Geometry check sheet. Reference: the model listing, model coordinates, mm. A direction names the side the tool comes from. Give positions to 0.01 mm unless a question says otherwise; leave off trailing zeros. Loops run counter-clockwise (first coordinate to the right, second up) from the corner with the lowest first, then second, coordinate; pieces in that order, holes last. Notation, with made-up numbers: (-30.75, -12) - (-15.75, -12) arc R22 ccw to (-15.75, 9) - close; hole circle Ø4 at (24, 54.25). An arc over 180 degrees is marked (long way). One line per question, with ' | ' between items. Start each with the question number.
from build123d import *

# Parameters (mm, degrees)
BOSS_EXTRUDE1_DEPTH = 13.125
SKETCH2_R           = 7
CUT_EXTRUDE1_DEPTH  = 106.5
SKETCH2_4_R         = 11.125
SKETCH2_4_R_2       = 7
CUT_EXTRUDE2_DEPTH  = 7
SKETCH4_R           = 4
BOSS_EXTRUDE3_DEPTH = 10
SKETCH5_R           = 6.5
BOSS_EXTRUDE4_DEPTH = 1
CIRPATTERN1_COUNT   = 2
CIRPATTERN1_ANGLE   = 45
SKETCH9_R           = 4
BOSS_EXTRUDE6_DEPTH = 20
CUT_EXTRUDE6_REACH  = 96.758
SKETCH10_R          = 1.5
SKETCH11_R          = 6.5
BOSS_EXTRUDE7_DEPTH = 13.5
SKETCH12_R          = 4
BOSS_EXTRUDE8_DEPTH = 13.75
SKETCH13_R          = 1.5
CUT_EXTRUDE7_DEPTH  = 13.75
SKETCH14_R          = 11.125
CUT_EXTRUDE8_DEPTH  = 17
SKETCH15_R          = 7
CUT_EXTRUDE9_DEPTH  = 1
SKETCH16_R          = 1.55
CUT_EXTRUDE10_DEPTH = 93.310955607


with BuildPart() as part:
    # Sketch1 → Boss-Extrude1 (new, symmetric)
    with BuildSketch(Plane(origin=(0, 0, 0), x_dir=(1, 0, 0), z_dir=(0, 1, 0))):
        Polygon((-49.25, 13.125), (-49.25, -13.125), (-49.25, -20.400017947), (-20.400017947, -49.25), (20.400017947, -49.25), (49.25, -20.400017947), (49.25, -13.125), (49.25, 13.125), (57.25, 13.125), (57.25, -23.713726446), (23.713726446, -57.25), (-23.713726446, -57.25), (-57.25, -23.713726446), (-57.25, 13.125), align=None)
    extrude(amount=BOSS_EXTRUDE1_DEPTH, both=True)

    # Sketch2 → Cut-Extrude1 (cut)
    with BuildSketch(Plane.ZY.offset(57.25)):
        with BuildLine():
            Line((-13.125, 13.125), (-13.125, 0))
            ThreePointArc((-13.125, 0), (-12.924585281, 2.284889562), (-12.329461667, 4.5))
            ThreePointArc((-12.329461667, 4.5), (-7.523400993, 10.7547228), (0, 13.125))
            Line((0, 13.125), (-13.125, 13.125))
        make_face()
        with BuildLine():
            ThreePointArc((-12.329461667, -4.5), (-12.924585281, -2.284889562), (-13.125, 0))
            Line((-13.125, 0), (-13.125, -13.125))
            Line((-13.125, -13.125), (0, -13.125))
            ThreePointArc((0, -13.125), (-7.523400993, -10.7547228), (-12.329461667, -4.5))
        make_face()
        Circle(SKETCH2_R)
        with BuildLine():
            ThreePointArc((-5.361902647, -4.5), (-6.577739678, -2.394439545), (-7, 0))
            Line((-7, 0), (-11.125, 0))
            ThreePointArc((-11.125, 0), (-10.88472093, -2.299668513), (-10.174262873, -4.5))
            Line((-10.174262873, -4.5), (-5.361902647, -4.5))
        make_face()
        with BuildLine():
            Line((-11.125, 0), (-7, 0))
            ThreePointArc((-7, 0), (-6.577739678, 2.394439545), (-5.361902647, 4.5))
            Line((-5.361902647, 4.5), (-10.174262873, 4.5))
            ThreePointArc((-10.174262873, 4.5), (-10.88472093, 2.299668513), (-11.125, 0))
        make_face()
        with BuildLine():
            ThreePointArc((-10.174262873, -4.5), (-10.88472093, -2.299668513), (-11.125, 0))
            Line((-11.125, 0), (-13.125, 0))
            ThreePointArc((-13.125, 0), (-12.924585281, -2.284889562), (-12.329461667, -4.5))
            Line((-12.329461667, -4.5), (-10.174262873, -4.5))
        make_face()
        with BuildLine():
            Line((-13.125, 0), (-11.125, 0))
            ThreePointArc((-11.125, 0), (-10.88472093, 2.299668513), (-10.174262873, 4.5))
            Line((-10.174262873, 4.5), (-12.329461667, 4.5))
            ThreePointArc((-12.329461667, 4.5), (-12.924585281, 2.284889562), (-13.125, 0))
        make_face()
    cut_extrude1 = extrude(amount=-CUT_EXTRUDE1_DEPTH, mode=Mode.SUBTRACT)

    # Sketch2_4 → Cut-Extrude2 (cut)
    with BuildSketch(Plane.ZY.offset(57.25)):
        Circle(SKETCH2_4_R)
        Circle(SKETCH2_4_R_2, mode=Mode.SUBTRACT)
    cut_extrude2 = extrude(amount=-CUT_EXTRUDE2_DEPTH, mode=Mode.SUBTRACT)

    # Mirror1: Cut-Extrude1, Cut-Extrude2 across plane
    add(cut_extrude1.mirror(Plane(origin=(0, 0, 0), x_dir=(0, 0, 1), z_dir=(1, 0, 0))), mode=Mode.SUBTRACT)
    add(cut_extrude2.mirror(Plane(origin=(0, 0, 0), x_dir=(0, 0, 1), z_dir=(1, 0, 0))), mode=Mode.SUBTRACT)

    # Sketch4 → Boss-Extrude3 (add)
    with BuildSketch(Plane(origin=(-40.481863223, 0, 40.481863223), x_dir=(0.7071067811865489, 0, 0.7071067811865461), z_dir=(-0.7071067811865461, 0, 0.7071067811865489))):
        with Locations(Location((0, 0, 0), (0, 0, 180))):
            Circle(SKETCH4_R)
    boss_extrude3 = extrude(amount=BOSS_EXTRUDE3_DEPTH)

    # Sketch5 → Boss-Extrude4 (add)
    with BuildSketch(Plane(origin=(-40.481863223, 0, 40.481863223), x_dir=(0.7071067811865489, 0, 0.7071067811865461), z_dir=(-0.7071067811865461, 0, 0.7071067811865489))):
        with Locations(Location((0, 0, 0), (0, 0, 180))):
            Circle(SKETCH5_R)
    boss_extrude4 = extrude(amount=BOSS_EXTRUDE4_DEPTH)

    # CirPattern1: Boss-Extrude3, Boss-Extrude4 ×2 about axis
    cirpattern1_axis = Axis((0, 14.4375, 0), (0, 1, 0))
    add([boss_extrude3.rotate(cirpattern1_axis, i * CIRPATTERN1_ANGLE / (CIRPATTERN1_COUNT - 1)) for i in range(1, CIRPATTERN1_COUNT)])
    add([boss_extrude4.rotate(cirpattern1_axis, i * CIRPATTERN1_ANGLE / (CIRPATTERN1_COUNT - 1)) for i in range(1, CIRPATTERN1_COUNT)])

    # Sketch9 → Boss-Extrude6 (add)
    with BuildSketch(Plane(origin=(-47.552931035, 0, 47.552931035), x_dir=(0.7071067811865489, 0, 0.7071067811865461), z_dir=(-0.7071067811865461, 0, 0.7071067811865489))):
        Circle(SKETCH9_R)
    extrude(amount=BOSS_EXTRUDE6_DEPTH)

    # Sketch10 → Cut-Extrude6 (cut, up to next)
    with BuildSketch(Plane(origin=(0, 4, 0), x_dir=(1, 0, 0), z_dir=(0, 1, 0)), mode=Mode.PRIVATE) as cut_extrude6_sk1:
        Polygon((-48.083261121, -53.74011537), (-53.74011537, -48.083261121), (-64.523493783, -58.866639534), (-58.866639534, -64.523493783), align=None)
    cut_extrude6_tool1 = extrude(cut_extrude6_sk1.sketch, amount=-CUT_EXTRUDE6_REACH, mode=Mode.PRIVATE) & part.part
    # Sketch10 → Cut-Extrude6 (cut, up to next)
    with BuildSketch(Plane(origin=(0, 4, 0), x_dir=(1, 0, 0), z_dir=(0, 1, 0)), mode=Mode.PRIVATE) as cut_extrude6_sk2:
        with Locations(Location((-48.083261121, -48.083261121, 0), (0, 0, 270))):
            Circle(SKETCH10_R)
    cut_extrude6_tool2 = extrude(cut_extrude6_sk2.sketch, amount=-CUT_EXTRUDE6_REACH, mode=Mode.PRIVATE) & part.part
    add(cut_extrude6_tool1.solids().sort_by_distance((-56.303377, 4, 56.303377))[0], mode=Mode.SUBTRACT)
    add(cut_extrude6_tool2.solids().sort_by_distance((-48.083261, 4, 48.083261))[0], mode=Mode.SUBTRACT)

    # Sketch11 → Boss-Extrude7 (add)
    with BuildSketch(Plane(origin=(40.481863223, 0, 40.481863223), x_dir=(0.7071067811865442, 0, -0.7071067811865508), z_dir=(0.7071067811865508, 0, 0.7071067811865442))):
        with Locations(Location((0, 0, 0), (0, 0, 180))):
            Circle(SKETCH11_R)
    extrude(amount=BOSS_EXTRUDE7_DEPTH)

    # Sketch12 → Boss-Extrude8 (add)
    with BuildSketch(Plane(origin=(50.027804769, 0, 50.027804769), x_dir=(0.7071067811865442, 0, -0.7071067811865508), z_dir=(0.7071067811865508, 0, 0.7071067811865442))):
        Circle(SKETCH12_R)
    extrude(amount=BOSS_EXTRUDE8_DEPTH)

    # Sketch13 → Cut-Extrude7 (cut)
    with BuildSketch(Plane(origin=(0, 4, 0), x_dir=(1, 0, 0), z_dir=(0, 1, 0))):
        with Locations(Location((56.922095886, -56.922095886, 0), (0, 0, 270))):
            Circle(SKETCH13_R)
    extrude(amount=-CUT_EXTRUDE7_DEPTH, mode=Mode.SUBTRACT)

    # Sketch14 → Cut-Extrude8 (cut)
    with BuildSketch(Plane.XY.offset(67.25)):
        Circle(SKETCH14_R)
    extrude(amount=-CUT_EXTRUDE8_DEPTH, mode=Mode.SUBTRACT)

    # Sketch15 → Cut-Extrude9 (cut)
    with BuildSketch(Plane.XY.offset(50.25)):
        Circle(SKETCH15_R)
    extrude(amount=-CUT_EXTRUDE9_DEPTH, mode=Mode.SUBTRACT)

    # Sketch16 → Cut-Extrude10 (cut, through all)
    with BuildSketch(Plane(origin=(0, 13.125, 0), x_dir=(1, 0, 0), z_dir=(0, 1, 0))):
        with Locations(Location((-53.25, -15, 0), (0, 0, 270))):
            Circle(SKETCH16_R)
        with Locations(Location((-53.25, -20.1, 0), (0, 0, 270))):
            Circle(SKETCH16_R)
    cut_extrude10 = extrude(amount=-CUT_EXTRUDE10_DEPTH, mode=Mode.SUBTRACT)

    # Mirror3: Cut-Extrude10 across plane
    add(cut_extrude10.mirror(Plane(origin=(0, 0, 0), x_dir=(0, 0, 1), z_dir=(1, 0, 0))), mode=Mode.SUBTRACT)


solid = part.part
(1) Section check B-B, the plane y = -8.75. Record the boundary of the cut face in (x, z), and give its area (3 significant figures).
(2) Material ranges on line 1 (X direction, y = -3.5, z = 15); line 2 (Z direction, x = 53.25, y = -5.5); line 3 (Y direction, x = 55.5, z = 0) (3 decimals), recorded low to high.
(3) Tool access check on faces 1 (the face through (52.42, 4.5, -10.35)), 2 (the face through (50.25, 0.2, 7.4)), 3 (the face through (-5, 6, 49.25)), 4 (the face through (57.25, 0, 13)), 5 (the face through (11, -3, 57.25)). Record the directions out of +Z, -Z, +X, -X, +Y, -Y that give a thin tool (end or side, any length) a straight path to the whole face; none if there is none.
(4) Section check D-D, the plane x = 19. Record the boundary of the cut face in (y, z) (3 decimals), and give its area (3 significant figures).
(5) Depth check by flat-ended pin: pin 1 Ø3.5 at (x, z) = (-53.5, -10) entering from -Y; pin 2 Ø6 at (x, y) = (48, -1.5) entering from -Z; pin 3 Ø10 at (x, y) = (2.5, 0.5) entering from +Z; pin 4 Ø2.5 at (x, z) = (-53.25, 15) entering from -Y. Enter the tip coordinate at first touch or a pass-through.
(6) Section check A-A, the plane x = 0. Record the boundary of the cut face in (y, z) (3 decimals), and give its area (4 significant figures).
(7) Mould release check, pull along X, two halves, no side actions. Record for faces 6 (the face through (-51.713, 0.184, 14.798)), 7 (the face through (-50.25, 0.2, 7.4)), 8 (the face through (-53.3, 10.7, -7.6)), 9 (the face through (-51.713, 0.184, 19.898)): pulls with the +X half, pulls with the -X half, needs draft (parallel to the pull), parting line crosses it, or undercut.
(8) Section check C-C, the plane z = 28. Record the boundary of the cut face in (x, y) (3 decimals), and give its area (3 significant figures).
Numbers:
1) outline: (-57.25, -9.78) - (-49.25, -9.78) - (-49.25, 20.4) - (-20.4, 49.25) - (20.4, 49.25) - (49.25, 20.4) - (49.25, -9.78) - (57.25, -9.78) - (57.25, -6.87) - (50.25, -6.87) - (50.25, 6.87) - (57.25, 6.87) - (57.25, 23.71) - (23.71, 57.25) - (6.87, 57.25) - (6.87, 50.25) - (-6.87, 50.25) - (-6.87, 57.25) - (-23.71, 57.25) - (-57.25, 23.71) - (-57.25, 6.87) - (-50.25, 6.87) - (-50.25, -6.87) - (-57.25, -6.87) - close; hole circle Ø3.1 at (-53.25, 15); hole circle Ø3.1 at (-53.25, 20.1); hole circle Ø3.1 at (53.25, 15); hole circle Ø3.1 at (53.25, 20.1) | area: 1,250 mm^2
2) line 1: -57.25 to -54.8, -51.7 to -49.25, 49.25 to 51.7, 54.8 to 57.25 | line 2: -11.92 to -9.67, 9.67 to 13.45, 16.55 to 18.55, 21.65 to 27.71 | line 3: -13.125 to -11.125, 11.125 to 13.125
3) face 1: -Z, +X, -X | face 2: +X | face 3: -Z, +Y, -Y | face 4: -Z, +X, +Y, -Y | face 5: +Z, -X, +Y, -Y
4) outline: (-13.125, 49.25) - (13.125, 49.25) - (13.125, 57.25) - (-13.125, 57.25) - close | area: 210 mm^2
5) pin 1: y = -10.21 | pin 2: z = 5.58 | pin 3: z = 50.25 | pin 4: through
6) outline: (-13.125, 49.25) - (-7, 49.25) - (-7, 50.25) - (-11.125, 50.25) - (-11.125, 57.25) - (-13.125, 57.25) - close; (7, 49.25) - (13.125, 49.25) - (13.125, 57.25) - (11.125, 57.25) - (11.125, 50.25) - (7, 50.25) - close | area: 40.25 mm^2
7) face 6: undercut | face 7: pulls with the -X half | face 8: needs draft | face 9: undercut
8) outline: (-52.964, -13.125) - (-41.65, -13.125) - (-41.65, 13.125) - (-52.964, 13.125) - close; (41.65, -13.125) - (52.964, -13.125) - (52.964, 13.125) - (41.65, 13.125) - close | area: 594 mm^2
